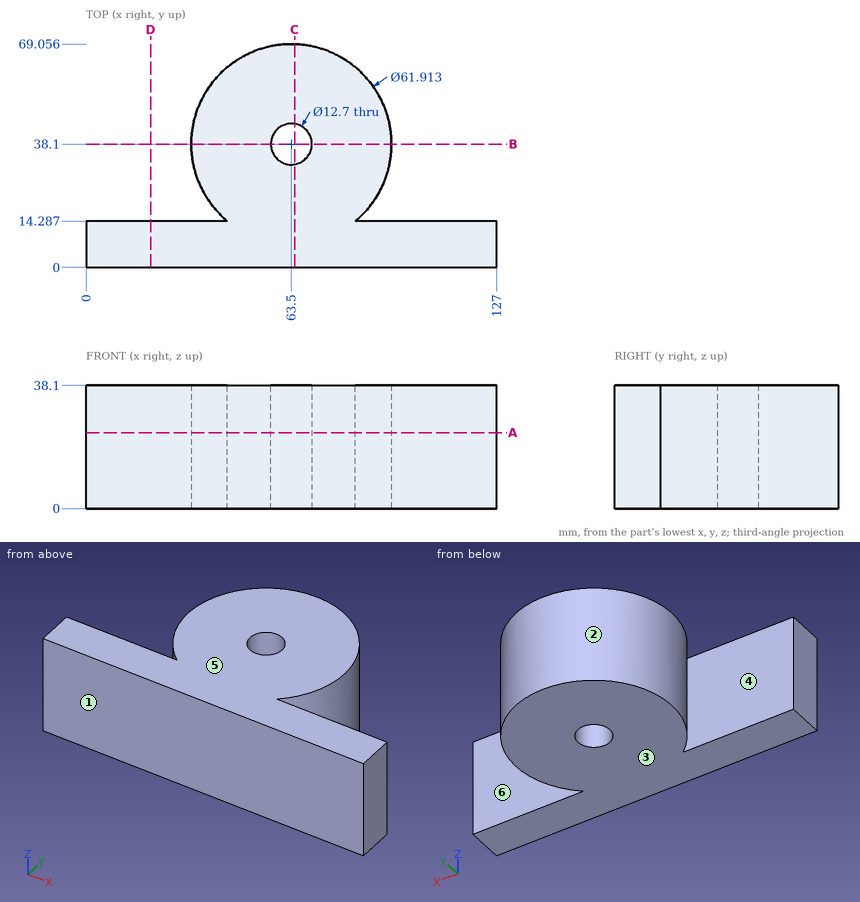
Answer from the drawing. Dimensions are ordinates in mm from the lowest x, y and z of the part. A direction names the side the tool comes from. Give positions to 0.01 mm unless a question says otherwise; leave off trailing zeros. Loops run counter-clockwise (first coordinate to the right, second up) from the corner with the lowest first, then second, coordinate; pieces in that order, holes last. Notation, with made-up numbers: (32.25, 55.25) - (77.25, 55.25) arc R30 ccw to (77.25, 92.25) - close; hole circle Ø11 at (-1.75, 42.5). An arc over 180 degrees is marked (long way). Answer as CSV lines item,"result". Start each with the question number.
Item 1: The mould has two halves that part along Y. Classify the marked faces 1, 2 and 3: +Y half, -Y half, draft (parallel to the pull), parting line (faces both ways), or undercut.
Item 2: A cutting plane is placed at A-A on z = 23.5. Determine the outline of the cut face in (x, y).
Item 3: Each of these flat-tipped pins is pushed along its axis until it touches: pin 1 (5 mm diameter, centred on y = 61.5, z = 16, fed in from -X) (1 decimal); pin 2 (11.5 mm diameter, centred on x = 18, z = 23, fed in from +Y); pin 3 (1 mm diameter, centred on x = 92, z = 6.5, fed in from +Y) (1 decimal). Where does it stop, or does it pass through?
Item 4: A cutting plane is placed at B-B on y = 38.1. Determine the outline of the cut face in (x, z).
Item 5: Find the intervals of material crossed by line 1 (Y direction, x = 63, z = 26); line 2 (Y direction, x = 63.5, z = 16); line 3 (X direction, y = 38.1, z = 30), in increasing order. Write a range as from..to.
Item 6: A cutting plane is placed at C-C on x = 64.5. Determine the outline of the cut face in (y, z).
Item 7: A cutting plane is placed at D-D on x = 20. Determine the outline of the cut face in (y, z), then the cut area to 3 significant figures.
Item 8: For the marked faces 4, 5 and 6, determine the directions among +Z, -Z, +X, -X, +Y, -Y from which every point of the face is accessible in a straight line to the end or side of a thin tool.
Found:
1,face 1,"-Y half"
1,face 2,"undercut"
1,face 3,"draft"
2,outline,"(0, 0) - (127, 0) - (127, 14.29) - (83.28, 14.29) arc R30.96 ccw (long way) to (43.72, 14.29) - (0, 14.29) - close; hole circle Ø12.7 at (63.5, 38.1)"
3,pin 1,"stops at x = 40.7"
3,pin 2,"stops at y = 14.29"
3,pin 3,"stops at y = 51.3"
4,outline,"(32.54, 0) - (57.15, 0) - (57.15, 38.1) - (32.54, 38.1) - close; (69.85, 0) - (94.46, 0) - (94.46, 38.1) - (69.85, 38.1) - close"
5,line 1,"y = 0..31.77, 44.43..69.05"
5,line 2,"y = 0..31.75, 44.45..69.06"
5,line 3,"x = 32.54..57.15, 69.85..94.46"
6,outline,"(0, 0) - (31.83, 0) - (31.83, 38.1) - (0, 38.1) - close; (44.37, 0) - (69.04, 0) - (69.04, 38.1) - (44.37, 38.1) - close"
7,outline,"(0, 0) - (14.29, 0) - (14.29, 38.1) - (0, 38.1) - close"
7,area,"544 mm^2"
8,face 4,"+Z, -Z, -X"
8,face 5,"+Z, +X, -X, +Y, -Y"
8,face 6,"+Z, -Z, +X"
